Source: CAD feature listing. Evaluate the final solid. Frame: model axes, mm. A direction names the side the tool comes from. Give positions to 0.01 mm unless a question says otherwise; leave off trailing zeros. Order: outer loops, then holes, each group sorted by start corner. A loop starts at its lowest first (then second) coordinate and runs counter-clockwise, first axis right, second up. Notation, with made-up numbers: M -27,-33 L -5,-33 A16 cw -5,-4 Z; hole C 19,28.25 d9. An arc over 180 degrees is marked long. Answer in a Markdown table with one row per item. Add a question column.
(1) Section query B-B, the plane x = 41. Return loops of the section in (y, z), plus the area to 3 significant figures.
(2) Section query C-C, the plane z = 0.6. Return loops of the section in (x, y), plus the area to 3 significant figures.
(3) Set-up query: faces 1 (the face through (49.195, 18.473, 1.268)), 2 (the face through (-49.195, 18.473, 1.268)), 3 (the face through (10, 11, 0)). Return all of +Z, -Z, +X, -X, +Y, -Y with unobstructed straight access to the full face (end or side cutting, diameter ignored); none if empty.
(4) Section query D-D, the plane y = -15.5. Return loops of the section in (x, z).
(5) Section query A-A, the plane y = -5. Return loops of the section in (x, z), plus the area to 3 significant figures.
(6) Pin query (flat end, axial travel): P1, Ø1, axis at y = -18.5, z = 2, coming from the +X side; P2, Ø4, axis at x = -4, y = 16, coming from the -Z side. Return the tip coordinate at first contact, or that it passes through.
(7) Material intervals for line 1 along Y through (x, z) = (24.5, 0.6); line 2 along Y through (x, z) = (-10, 1.25); line 3 along X through (y, z) = (-1, 2.05), sorted ascending.
(8) Mould query, pull axis Y, two halves, no side actions, for faces 4 (the face through (12.932, -5.362, 1.232)), 5 (the face through (-41, -25, 1)), 6 (the face through (-41, 25, 1)). Classes: pulls with the +Y half, pulls with the -Y half, needs draft (parallel to the pull), parting line crosses it, or undercut.
from build123d import *

# Parameters (mm, degrees)
SKETCH_R    = 14
SKETCH_R_2  = 3
PAD_DEPTH   = 2.5
FILLET_R    = 3.5
FILLET001_R = 1


with BuildPart() as part:
    # Sketch → Pad (new body)
    with BuildSketch(Plane.XY):
        with BuildLine():
            Line((-50, 25), (-50, 17.5))
            ThreePointArc((-50, -17.5), (-32.5, 0), (-50, 17.5))
            Line((-50, -17.5), (-50, -25))
            Line((-50, -25), (-35.336948, -25))
            ThreePointArc((35.336948, -25), (0, -22.49), (-35.336948, -25))
            Line((35.336948, -25), (50, -25))
            Line((50, -25), (50, -17.5))
            ThreePointArc((50, 17.5), (32.5, 0), (50, -17.5))
            Line((50, 17.5), (50, 25))
            Line((50, 25), (35.336948, 25))
            ThreePointArc((-35.336948, 25), (0, 22.49), (35.336948, 25))
            Line((-35.336948, 25), (-50, 25))
        make_face()
        Circle(SKETCH_R, mode=Mode.SUBTRACT)
        with Locations((25.44788, 17.156958)):
            Circle(SKETCH_R_2, mode=Mode.SUBTRACT)
    extrude(amount=PAD_DEPTH)

    # Fillet
    fillet_edges = [part.edges().sort_by_distance(p)[0] for p in [
        (-50, -25, 1.25),
        (50, -25, 1.25),
        (50, -17.5, 1.25),
        (50, 25, 1.25),
        (50, 17.5, 1.25),
        (-50, 17.5, 1.25),
        (-50, 25, 1.25),
        (-50, -17.5, 1.25),
    ]]
    fillet(fillet_edges, radius=FILLET_R)

    # Fillet001
    fillet001_edges = [part.edges().sort_by_distance(p)[0] for p in [
        (35.336948, 25, 1.25),
        (-35.336948, 25, 1.25),
        (-35.336948, -25, 1.25),
        (35.336948, -25, 1.25),
    ]]
    fillet(fillet001_edges, radius=FILLET001_R)


solid = part.part
Values follow:
| question | item | result |
|---|---|---|
| 1 | outline | M -25,0 L -15.01,0 L -15.01,2.5 L -25,2.5 Z; M 15.01,0 L 25,0 L 25,2.5 L 15.01,2.5 Z |
| 1 | area | 50.0 mm² |
| 2 | outline | M -50,-21.5 A3.5 ccw -46.5,-25 L -35.41,-25 A1 ccw -35.27,-24.99 A250 cw 35.27,-24.99 A1 ccw 35.41,-25 L 46.5,-25 A3.5 ccw 50,-21.5 L 50,-20.71 A3.5 ccw 47.08,-17.26 A17.5 cw 47.08,17.26 A3.5 ccw 50,20.71 L 50,21.5 A3.5 ccw 46.5,25 L 35.41,25 A1 ccw 35.27,24.99 A250 cw -35.27,24.99 A1 ccw -35.41,25 L -46.5,25 A3.5 ccw -50,21.5 L -50,20.71 A3.5 ccw -47.08,17.26 A17.5 cw -47.08,-17.26 A3.5 ccw -50,-20.71 Z; hole C 0,0 d28; hole C 25.45,17.16 d6 |
| 2 | area | 3,140 mm² |
| 3 | face 1 | +Z, -Z, +X |
| 3 | face 2 | +Z, -Z, -X |
| 3 | face 3 | -Z, +X, -X, +Y, -Y |
| 4 | outline | M -41.88,0 L 41.88,0 L 41.88,2.5 L -41.88,2.5 Z |
| 5 | outline | M -33.23,0 L -13.08,0 L -13.08,2.5 L -33.23,2.5 Z; M 13.08,0 L 33.23,0 L 33.23,2.5 L 13.08,2.5 Z |
| 5 | area | 101 mm² |
| 6 | P1 | stops at x = 49.56 |
| 6 | P2 | stops at z = 0 |
| 7 | line 1 | y = -23.69 to 14.31, 20 to 23.69 |
| 7 | line 2 | y = -22.69 to -9.8, 9.8 to 22.69 |
| 7 | line 3 | x = -32.53 to -13.96, 13.96 to 32.53 |
| 8 | face 4 | undercut |
| 8 | face 5 | pulls with the -Y half |
| 8 | face 6 | pulls with the +Y half |
